from build123d import *

# Parameters (mm, degrees)
ESQUISSE1_R             = 5
BOSS_EXTRU_1_DEPTH      = 15
ESQUISSE2_W             = 30
ESQUISSE2_H             = 12.881717487
ENL_V_MAT_EXTRU_1_DEPTH = 15
ESQUISSE3_W             = 20
ESQUISSE3_H             = 15
ENL_V_MAT_EXTRU_2_DEPTH = 15
ESQUISSE5_R             = 15
BOSS_EXTRU_2_DEPTH      = 37.5


with BuildPart() as part:
    # Esquisse1 → Boss.-Extru.1 (new body)
    with BuildSketch(Plane.XY):
        with BuildLine():
            Line((-160.494422558, 41.644450698), (-27.47211279, 79.650824917))
            ThreePointArc((-27.47211279, 79.650824917), (0, 83.498430153), (27.47211279, 79.650824917))
            Line((27.47211279, 79.650824917), (160.494422558, 41.644450698))
            ThreePointArc((160.494422558, 41.644450698), (170.966972962, 34.457882008), (175, 22.413971745))
            Line((175, 22.413971745), (175, -17.5))
            ThreePointArc((175, -17.5), (169.142135624, -31.642135624), (155, -37.5))
            Line((155, -37.5), (-155, -37.5))
            ThreePointArc((-155, -37.5), (-169.142135624, -31.642135624), (-175, -17.5))
            Line((-175, -17.5), (-175, 22.413971745))
            ThreePointArc((-175, 22.413971745), (-170.966972962, 34.457882008), (-160.494422558, 41.644450698))
        make_face()
        with Locations((0, 68.16509682)):
            Circle(ESQUISSE1_R, mode=Mode.SUBTRACT)
    extrude(amount=BOSS_EXTRU_1_DEPTH)

    # Esquisse2 → Enlèv. mat.-Extru.1 (cut)
    with BuildSketch(Plane.XY.offset(15)):
        Polygon((95, -37.5), (115, -37.5), (125, -37.5), (135, -37.5), (135, -22.5), (125, -22.5), (125, -13.549697849), (132.5, -13.549697849), (132.5, -3.549697849), (125, -3.549697849), (125, 7.276030806), (115, 7.276030806), (115, -3.549697849), (107.5, -3.549697849), (107.5, -13.549697849), (115, -13.549697849), (115, -22.5), (95, -22.5), align=None)
        with Locations((30, -31.059141256)):
            Rectangle(ESQUISSE2_W, ESQUISSE2_H)
        with Locations((-30, -31.059141256)):
            Rectangle(ESQUISSE2_W, ESQUISSE2_H)
        Polygon((-115, -37.5), (-95, -37.5), (-95, -22.5), (-115, -22.5), (-115, -13.549697849), (-107.5, -13.549697849), (-107.5, -3.549697849), (-115, -3.549697849), (-115, 7.276030806), (-125, 7.276030806), (-125, -3.549697849), (-132.5, -3.549697849), (-132.5, -13.549697849), (-125, -13.549697849), (-125, -22.5), (-135, -22.5), (-135, -37.5), (-125, -37.5), align=None)
    extrude(amount=-ENL_V_MAT_EXTRU_1_DEPTH, mode=Mode.SUBTRACT)

    # Esquisse3 → Enlèv. mat.-Extru.2 (cut)
    with BuildSketch(Plane(origin=(0, 0, 0), x_dir=(-1, 0, 0), z_dir=(0, 0, -1))):
        with Locations((145, -30)):
            Rectangle(ESQUISSE3_W, ESQUISSE3_H)
        with Locations((-145, -30)):
            Rectangle(ESQUISSE3_W, ESQUISSE3_H)
    extrude(amount=-ENL_V_MAT_EXTRU_2_DEPTH, mode=Mode.SUBTRACT)

    # Esquisse5 → Boss.-Extru.2 (add)
    with BuildSketch(Plane.XY.offset(15)):
        with Locations((0.685853551, 68.16509682)):
            Circle(ESQUISSE5_R)
    extrude(amount=BOSS_EXTRU_2_DEPTH)


solid = part.part
Model file for the job. Use its own axes, mm. A direction names the side the tool comes from. Give positions to 0.01 mm unless a question says otherwise; leave off trailing zeros. Loops run counter-clockwise (first coordinate to the right, second up) from the corner with the lowest first, then second, coordinate; pieces in that order, holes last.
Item 1: Drill centre lines: line 1 along X through (y, z) = (-19, 2.5); line 2 along X through (y, z) = (-11.5, 5); line 3 along Y through (x, z) = (0, 9). Where is each one in solid material? Low to high.
Check values:
line 1: x = -174.94 to -125, -115 to 115, 125 to 174.94
line 2: x = -175 to -132.5, -107.5 to 107.5, 132.5 to 175
line 3: y = -37.5 to 63.17, 73.17 to 83.5
Item 2: Slice it at C-C (x = 9). Write the cut outline in (y, z).
Check values:
outline: (-37.5, 0) - (83.09, 0) - (83.09, 15) - (80.65, 15) - (80.65, 52.5) - (55.68, 52.5) - (55.68, 15) - (-37.5, 15) - close
Item 3: Slice it at D-D (y = 46). Write the cut outline in (x, z).
Check values:
outline: (-145.25, 0) - (145.25, 0) - (145.25, 15) - (-145.25, 15) - close
Item 4: Drop flat-ended pins along their axis: P1, Ø16.5, axis at y = -31.5, z = 6, coming from the -X side; P2, Ø12, axis at x = -77.5, y = -2.5, coming from the -Z side; P3, Ø2, axis at x = -128.5, z = 7.5, coming from the +Y side; P4, Ø4, axis at y = -31, z = 10, coming from the +X side. Give the stop position or say it passes through.
Check values:
P1: stops at x = -174.16
P2: stops at z = 0
P3: stops at y = 51.07
P4: stops at x = 171.36
Item 5: Which spindle directions (+Z, -Z, +X, -X, +Y, -Y) get a long thin tool onto all of the face, cutting with end or side? Do faces 1 (the face through (107.5, -8, 8)), 2 (the face through (115, -18, 8)), 3 (the face through (0, 68, 15)), 4 (the face through (170.86, 34.6, 7.4)). Say none if no direction does.
Check values:
face 1: +Z, -Z
face 2: +Z, -Z, -Y
face 3: -Z
face 4: +Z, -Z, +X, +Y
Item 6: Mould opens along X. For faces 5 (the face through (-94.914, 60.382, 7.395)), 6 (the face through (2, 10, 15)), 7 (the face through (132.5, -9, 8)) say: +X half, -X half, draft (parallel to the pull), parting line (faces both ways), or undercut.
Check values:
face 5: -X half
face 6: draft
face 7: undercut
Item 7: Slice it at A-A (y = -29.5). Write the cut outline in (x, z), plus the area to 3 significant figures.
Check values:
outline: (-171, 0) - (-155, 0) - (-155, 15) - (-171, 15) - close; (-95, 0) - (-45, 0) - (-45, 15) - (-95, 15) - close; (-15, 0) - (15, 0) - (15, 15) - (-15, 15) - close; (45, 0) - (95, 0) - (95, 15) - (45, 15) - close; (155, 0) - (171, 0) - (171, 15) - (155, 15) - close
area: 2,430 mm2
Item 8: Slice it at B-B (y = 3). Write the cut outline in (x, z), plus the area to 3 significant figures.
Check values:
outline: (-175, 0) - (-125, 0) - (-125, 15) - (-175, 15) - close; (-115, 0) - (115, 0) - (115, 15) - (-115, 15) - close; (125, 0) - (175, 0) - (175, 15) - (125, 15) - close
area: 4,950 mm2
